from build123d import *

# Parameters (mm, degrees)
SKETCH1_W             = 10
SKETCH1_H             = 10
BOSS_EXTRUDE1_DEPTH   = 400
BOSS_EXTRUDE1_2_DEPTH = 400
BOSS_EXTRUDE1_3_DEPTH = 400
BOSS_EXTRUDE1_4_DEPTH = 400
SKETCH2_W             = 10
SKETCH2_H             = 10
BOSS_EXTRUDE2_DEPTH   = 400
SKETCH3_W             = 220
SKETCH3_H             = 220
BOSS_EXTRUDE3_DEPTH   = 5
SKETCH4_W             = 10
SKETCH4_H             = 292.424434456
BOSS_EXTRUDE4_DEPTH   = 200
SKETCH5_R             = 11.390876375
CUT_EXTRUDE1_DEPTH    = 200


with BuildPart() as part:
    # Sketch1 → Boss-Extrude1 (new body)
    with BuildSketch(Plane(origin=(0, 0, 0), x_dir=(1, 0, 0), z_dir=(0, 1, 0))):
        with Locations((-105, 105)):
            Rectangle(SKETCH1_W, SKETCH1_H)
    extrude(amount=BOSS_EXTRUDE1_DEPTH)



with BuildPart() as body_2:
    # Sketch1 → Boss-Extrude1 2 (new body)
    with BuildSketch(Plane(origin=(0, 0, 0), x_dir=(1, 0, 0), z_dir=(0, 1, 0))):
        with Locations((105, 105)):
            Rectangle(SKETCH1_W, SKETCH1_H)
    extrude(amount=BOSS_EXTRUDE1_2_DEPTH)


with BuildPart() as body_3:
    # Sketch1 → Boss-Extrude1 3 (new body)
    with BuildSketch(Plane(origin=(0, 0, 0), x_dir=(1, 0, 0), z_dir=(0, 1, 0))):
        with Locations((105, -105)):
            Rectangle(SKETCH1_W, SKETCH1_H)
    extrude(amount=BOSS_EXTRUDE1_3_DEPTH)


with BuildPart() as body_4:
    # Sketch1 → Boss-Extrude1 4 (new body)
    with BuildSketch(Plane(origin=(0, 0, 0), x_dir=(1, 0, 0), z_dir=(0, 1, 0))):
        with Locations((-105, -105)):
            Rectangle(SKETCH1_W, SKETCH1_H)
    extrude(amount=BOSS_EXTRUDE1_4_DEPTH)


with BuildPart() as part_1:
    add(part.part)

    add(body_2.part)  # Boss-Extrude2 merges body 2
    # Sketch2 → Boss-Extrude2 (add)
    with BuildSketch(Plane(origin=(0, 400, 0), x_dir=(1, 0, 0), z_dir=(0, 1, 0))):
        with Locations((105, 105)):
            Rectangle(SKETCH2_W, SKETCH2_H)
        with Locations((-105, 105)):
            Rectangle(SKETCH2_W, SKETCH2_H)
    extrude(amount=BOSS_EXTRUDE2_DEPTH)


    add(body_3.part)  # Boss-Extrude3 merges body 3

    add(body_4.part)  # Boss-Extrude3 merges body 4
    # Sketch3 → Boss-Extrude3 (add)
    with BuildSketch(Plane(origin=(0, 400, 0), x_dir=(1, 0, 0), z_dir=(0, 1, 0))):
        Rectangle(SKETCH3_W, SKETCH3_H)
    extrude(amount=BOSS_EXTRUDE3_DEPTH)

    # Sketch4 → Boss-Extrude4 (add)
    with BuildSketch(Plane(origin=(-100, 0, 0), x_dir=(0, 0, -1), z_dir=(1, 0, 0))):
        with Locations((105, 642.632960166)):
            Rectangle(SKETCH4_W, SKETCH4_H)
    extrude(amount=BOSS_EXTRUDE4_DEPTH)

    # Sketch5 → Cut-Extrude1 (cut)
    with BuildSketch(Plane.XY.offset(-100)):
        with Locations((-78.87817112, 766.657257613)):
            Circle(SKETCH5_R)
        with Locations((-51.294465102, 766.657257613)):
            Circle(SKETCH5_R)
        with Locations((-24.073702585, 766.657257613)):
            Circle(SKETCH5_R)
        with Locations((1.695285931, 766.657257613)):
            Circle(SKETCH5_R)
        with Locations((27.464274447, 766.657257613)):
            Circle(SKETCH5_R)
        with Locations((53.233262963, 766.657257613)):
            Circle(SKETCH5_R)
        with Locations((79.728138479, 766.657257613)):
            Circle(SKETCH5_R)
        with Locations((79.728138479, 721.652263585)):
            Circle(SKETCH5_R)
        with Locations((53.233262963, 721.652263585)):
            Circle(SKETCH5_R)
        with Locations((27.464274447, 721.652263585)):
            Circle(SKETCH5_R)
        with Locations((1.695285931, 721.652263585)):
            Circle(SKETCH5_R)
        with Locations((-24.073702585, 721.652263585)):
            Circle(SKETCH5_R)
        with Locations((-51.294465102, 721.652263585)):
            Circle(SKETCH5_R)
        with Locations((-78.87817112, 721.652263585)):
            Circle(SKETCH5_R)
        with Locations((-78.87817112, 604.784456512)):
            Circle(SKETCH5_R)
        with Locations((-51.294465102, 604.784456512)):
            Circle(SKETCH5_R)
        with Locations((-24.073702585, 604.784456512)):
            Circle(SKETCH5_R)
        with Locations((1.695285931, 604.784456512)):
            Circle(SKETCH5_R)
        with Locations((27.464274447, 604.784456512)):
            Circle(SKETCH5_R)
        with Locations((53.233262963, 604.784456512)):
            Circle(SKETCH5_R)
        with Locations((79.728138479, 604.784456512)):
            Circle(SKETCH5_R)
        with Locations((79.728138479, 559.779462484)):
            Circle(SKETCH5_R)
        with Locations((53.233262963, 559.779462484)):
            Circle(SKETCH5_R)
        with Locations((27.464274447, 559.779462484)):
            Circle(SKETCH5_R)
        with Locations((1.695285931, 559.779462484)):
            Circle(SKETCH5_R)
        with Locations((-24.073702585, 559.779462484)):
            Circle(SKETCH5_R)
        with Locations((-51.294465102, 559.779462484)):
            Circle(SKETCH5_R)
        with Locations((-78.87817112, 559.779462484)):
            Circle(SKETCH5_R)
    extrude(amount=-CUT_EXTRUDE1_DEPTH, mode=Mode.SUBTRACT)


solid = part_1.part
Read the model definition and answer for the solid it produces. Units are mm, in the model's axes. Coordinates: 2 decimals unless noted, no trailing zeros. Write each loop counter-clockwise with the first axis right and the second up, starting at its lowest first coordinate (ties: lowest second). Pieces come first, ordered by that corner, then holes. Notation, with made-up numbers: (84.5, 47.25) - (89.5, 47.25) arc R25 cw to (89.5, 67.25) - close; hole circle Ø11 at (-2, 83.5). An arc over 180 degrees is marked (long way). One line per question, with ' | ' between items.
Q1. Find section D-D, the plane z = -67.5. Write down the section's boundary in (x, y).
Result set:
outline: (-110, 400) - (110, 400) - (110, 405) - (-110, 405) - close
Q2. Find section C-C, the plane x = -77. Write down the section's boundary in (y, z), plus the area to 3 significant figures.
Result set:
outline: (400, -110) - (405, -110) - (405, 110) - (400, 110) - close; (496.42, -110) - (548.54, -110) - (548.54, -100) - (496.42, -100) - close; (571.01, -110) - (593.55, -110) - (593.55, -100) - (571.01, -100) - close; (616.02, -110) - (710.42, -110) - (710.42, -100) - (616.02, -100) - close; (732.89, -110) - (755.42, -110) - (755.42, -100) - (732.89, -100) - close; (777.89, -110) - (788.85, -110) - (788.85, -100) - (777.89, -100) - close | area: 3,130 mm^2
Q3. Find section B-B, the plane x = 76. Write down the section's boundary in (y, z).
Result set:
outline: (400, -110) - (405, -110) - (405, 110) - (400, 110) - close; (496.42, -110) - (549.02, -110) - (549.02, -100) - (496.42, -100) - close; (570.54, -110) - (594.02, -110) - (594.02, -100) - (570.54, -100) - close; (615.55, -110) - (710.89, -110) - (710.89, -100) - (615.55, -100) - close; (732.42, -110) - (755.89, -110) - (755.89, -100) - (732.42, -100) - close; (777.42, -110) - (788.85, -110) - (788.85, -100) - (777.42, -100) - close
Q4. Each of these flat-tipped pins is pushed along its axis until it touches: P1, Ø8, axis at x = 28.5, z = -105, coming from the -Y side; P2, Ø5, axis at x = 4, y = 545.5, coming from the +Z side. Where does it stop, or does it pass through?
Result set:
P1: y = 400 | P2: z = -100
Q5. Determine the mould class of faces 1 (the flat face through (110, 339, -105)), 2 (the cylindrical face through (-0.77, 548.66, -104.93)), 3 (the flat face through (-110, 339, -105)) for opening direction X: +X half, -X half, draft (parallel to the pull), parting line (faces both ways), or undercut.
Result set:
face 1: +X half | face 2: undercut | face 3: -X half
Q6. Consider L1, parallel to Y at x = 89.5, z = 3.5; L2, parallel to Z at x = -40.5, y = 569.5. Determine where each line is inside the solid, lowest interval first. Write a range as [from, to].
Result set:
L1: [400, 405] | L2: [-110, -100]
Q7. Find section A-A, the plane y = 76.5. Write down the section's boundary in (x, z).
Result set:
outline: (-110, -110) - (-100, -110) - (-100, -100) - (-110, -100) - close; (-110, 100) - (-100, 100) - (-100, 110) - (-110, 110) - close; (100, -110) - (110, -110) - (110, -100) - (100, -100) - close; (100, 100) - (110, 100) - (110, 110) - (100, 110) - close
